Geometry: final body of the model. Coordinates: model frame, mm. Face numbers are marked on the shaded views. A direction names the side the tool comes from. Coordinates: 2 decimals unless noted, no trailing zeros. Write each loop counter-clockwise with the first axis right and the second up, starting at its lowest first coordinate (ties: lowest second). Pieces come first, ordered by that corner, then holes. Notation, with made-up numbers: (19.5, 27) -> (35.5, 27) arc R13 ccw to (35.5, 36) -> close; hole circle Ø5 at (0.5, 48). An arc over 180 degrees is marked (long way). One line per item, written item: value.
```python
from build123d import *

# Parameters (mm, degrees)
SKETCH1_R               = 10
BOSS_EXTRUDE1_DEPTH     = 65
CUT_EXTRUDE1_DEPTH      = 18
CUT_EXTRUDE1_DEPTH_BACK = 16
SKETCH2_R               = 2
SKETCH5_R               = 15
BOSS_EXTRUDE3_DEPTH     = 5
SCALE1_SCALE            = 0.5


with BuildPart() as part:
    # Sketch1 → Boss-Extrude1 (new body)
    with BuildSketch(Plane.XY):
        Circle(SKETCH1_R)
    extrude(amount=BOSS_EXTRUDE1_DEPTH)

    # Sketch2 → Cut-Extrude1 (cut, two sides: drawn at the far end of the back side and taken through both)
    with BuildSketch(Plane(origin=(0, 0, 0), x_dir=(0, 0, -1), z_dir=(1, 0, 0)).offset(-CUT_EXTRUDE1_DEPTH_BACK)):
        with Locations(Location((-61.5, 0, 0), (0, 0, 180))):
            Circle(SKETCH2_R)
    extrude(amount=CUT_EXTRUDE1_DEPTH + CUT_EXTRUDE1_DEPTH_BACK, mode=Mode.SUBTRACT)

    # Sketch5 → Boss-Extrude3 (add)
    with BuildSketch(Plane(origin=(0, 0, 0), x_dir=(-1, 0, 0), z_dir=(0, 0, -1))):
        Circle(SKETCH5_R)
    extrude(amount=-BOSS_EXTRUDE3_DEPTH)


with BuildPart() as part_1:
    # Scale1: scaled about (0, 0, 0)
    add(part.part.scale(SCALE1_SCALE))


solid = part_1.part
```
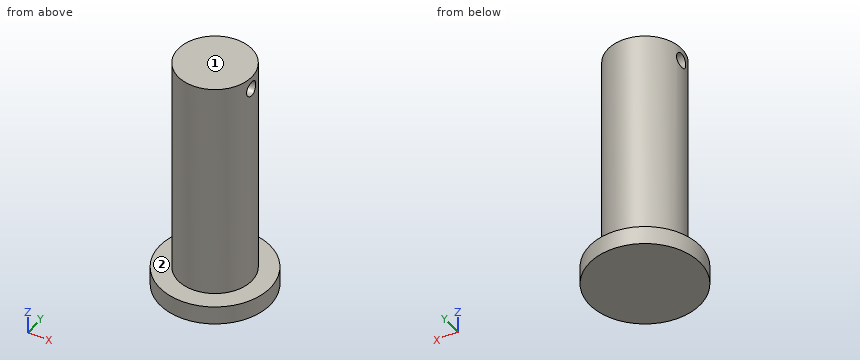
(1) Line query: line 1 (Y direction, x = 0, z = 30.75); line 2 (Z direction, x = 0, y = -5.75); line 3 (Y direction, x = -2.25, z = 30.75). Output: solid intervals per line, ascending. Write a range as [from, to].
Responses:
line 1: y = [-5, -1], [1, 5]
line 2: z = [0, 2.5]
line 3: y = [-4.47, -1], [1, 4.47]
(2) First-contact query: pin 1 (5 mm diameter, centred on x = 5.5, z = 20.5, fed in from -Y); pin 2 (3 mm diameter, centred on x = -5, y = -5, fed in from +Z); pin 3 (4 mm diameter, centred on x = 3, y = -4.5, fed in from +Z); pin 4 (1 mm diameter, centred on y = -2.5, z = 8.5, fed in from -X). Flat tips, straight axial feed; report the tip coordinate or a pass-through.
Responses:
pin 1: stops at y = -4
pin 2: stops at z = 2.5
pin 3: stops at z = 32.5
pin 4: stops at x = -4.58
(3) Reachability of the marked faces 1 and 2 from +Z, -Z, +X, -X, +Y, -Y: full face, straight path, thin tool, end or side. Return the list, or none.
Responses:
face 1: +Z, +X, -X, +Y, -Y
face 2: +Z
(4) Section D-D (z = 30.75). Return the cut outline in (x, y).
Responses:
outline: (-4.9, -1) arc R5 ccw to (4.9, -1) -> close; (-4.9, 1) -> (4.9, 1) arc R5 ccw to start
(5) Section C-C (z = 5.5). Return the cut outline in (x, y).
Responses:
outline: circle Ø10 at (0, 0)
(6) Section A-A (y = 0). Return the cut outline in (x, z).
Responses:
outline: (-7.5, 0) -> (7.5, 0) -> (7.5, 2.5) -> (5, 2.5) -> (5, 29.75) -> (-5, 29.75) -> (-5, 2.5) -> (-7.5, 2.5) -> close; (-5, 31.75) -> (5, 31.75) -> (5, 32.5) -> (-5, 32.5) -> close
(7) Section B-B (x = 0). Return the cut outline in (y, z).
Responses:
outline: (-7.5, 0) -> (7.5, 0) -> (7.5, 2.5) -> (5, 2.5) -> (5, 32.5) -> (-5, 32.5) -> (-5, 2.5) -> (-7.5, 2.5) -> close; hole circle Ø2 at (0, 30.75)
